```python
from build123d import *

# Parameters (mm, degrees)
SKETCH1_R               = 9.05
BOSS_EXTRUDE1_DEPTH     = 1.5
SKETCH2_R               = 7.83
BOSS_EXTRUDE2_DEPTH     = 11
CUT_EXTRUDE1_START      = -11
CUT_EXTRUDE1_DEPTH      = 11
SKETCH3_R               = 9.05
BOSS_EXTRUDE3_DEPTH     = 1.5
SKETCH5_R               = 6
BOSS_EXTRUDE4_DEPTH     = 9
SKETCH6_R               = 2.5
CUT_EXTRUDE2_DEPTH      = 27.321189183
CUT_EXTRUDE3_DEPTH      = 27.321189183
CUT_EXTRUDE3_DEPTH_BACK = 27.321189183
SKETCH7_R               = 1.5
FILLET1_R               = 0.2


with BuildPart() as part:
    # Sketch1 → Boss-Extrude1 (new body)
    with BuildSketch(Plane(origin=(0, 0, 0), x_dir=(1, 0, 0), z_dir=(0, 1, 0))):
        with Locations(Location((0, 0, 0), (0, 0, 270))):
            Circle(SKETCH1_R)
    extrude(amount=BOSS_EXTRUDE1_DEPTH)

    # Sketch2 → Boss-Extrude2 (add)
    with BuildSketch(Plane(origin=(0, 1.5, 0), x_dir=(1, 0, 0), z_dir=(0, 1, 0))):
        with Locations(Location((0, 0, 0), (0, 0, 270))):
            Circle(SKETCH2_R)
    extrude(amount=BOSS_EXTRUDE2_DEPTH)

    # Sketch4 → Cut-Extrude1 (cut)
    with BuildSketch(Plane(origin=(0, 12.5, 0), x_dir=(1, 0, 0), z_dir=(0, 1, 0)).offset(CUT_EXTRUDE1_START)):
        with BuildLine():
            Line((-1.095041255, 6.913818384), (-1.224881861, 7.733599707))
            ThreePointArc((-1.224881861, 7.733599707), (0, 7.83), (1.224881861, 7.733599707))
            Line((1.224881861, 7.733599707), (1.095041255, 6.913818384))
            ThreePointArc((1.095041255, 6.913818384), (0, 7), (-1.095041255, 6.913818384))
        make_face()
        with BuildLine():
            Line((3.177933498, 6.237045669), (3.554745613, 6.976581084))
            ThreePointArc((3.554745613, 6.976581084), (4.602358525, 6.334603066), (5.536646097, 5.536646097))
            Line((5.536646097, 5.536646097), (4.949747468, 4.949747468))
            ThreePointArc((4.949747468, 4.949747468), (4.114496766, 5.663118961), (3.177933498, 6.237045669))
        make_face()
        with BuildLine():
            Line((6.237045669, 3.177933498), (6.976581084, 3.554745613))
            ThreePointArc((6.976581084, 3.554745613), (7.446772523, 2.419603066), (7.733599707, 1.224881861))
            Line((7.733599707, 1.224881861), (6.913818384, 1.095041255))
            ThreePointArc((6.913818384, 1.095041255), (6.657395614, 2.163118961), (6.237045669, 3.177933498))
        make_face()
        with BuildLine():
            Line((6.913818384, -1.095041255), (7.733599707, -1.224881861))
            ThreePointArc((7.733599707, -1.224881861), (7.446772523, -2.419603066), (6.976581084, -3.554745613))
            Line((6.976581084, -3.554745613), (6.237045669, -3.177933498))
            ThreePointArc((6.237045669, -3.177933498), (6.657395614, -2.163118961), (6.913818384, -1.095041255))
        make_face()
        with BuildLine():
            Line((4.949747468, -4.949747468), (5.536646097, -5.536646097))
            ThreePointArc((5.536646097, -5.536646097), (4.602358525, -6.334603066), (3.554745613, -6.976581084))
            Line((3.554745613, -6.976581084), (3.177933498, -6.237045669))
            ThreePointArc((3.177933498, -6.237045669), (4.114496766, -5.663118961), (4.949747468, -4.949747468))
        make_face()
        with BuildLine():
            Line((1.095041255, -6.913818384), (1.224881861, -7.733599707))
            ThreePointArc((1.224881861, -7.733599707), (0, -7.83), (-1.224881861, -7.733599707))
            Line((-1.224881861, -7.733599707), (-1.095041255, -6.913818384))
            ThreePointArc((-1.095041255, -6.913818384), (0, -7), (1.095041255, -6.913818384))
        make_face()
        with BuildLine():
            Line((-3.177933498, -6.237045669), (-3.554745613, -6.976581084))
            ThreePointArc((-3.554745613, -6.976581084), (-4.602358525, -6.334603066), (-5.536646097, -5.536646097))
            Line((-5.536646097, -5.536646097), (-4.949747468, -4.949747468))
            ThreePointArc((-4.949747468, -4.949747468), (-4.114496766, -5.663118961), (-3.177933498, -6.237045669))
        make_face()
        with BuildLine():
            Line((-6.237045669, -3.177933498), (-6.976581084, -3.554745613))
            ThreePointArc((-6.976581084, -3.554745613), (-7.446772523, -2.419603066), (-7.733599707, -1.224881861))
            Line((-7.733599707, -1.224881861), (-6.913818384, -1.095041255))
            ThreePointArc((-6.913818384, -1.095041255), (-6.657395614, -2.163118961), (-6.237045669, -3.177933498))
        make_face()
        with BuildLine():
            Line((-6.913818384, 1.095041255), (-7.733599707, 1.224881861))
            ThreePointArc((-7.733599707, 1.224881861), (-7.446772523, 2.419603066), (-6.976581084, 3.554745613))
            Line((-6.976581084, 3.554745613), (-6.237045669, 3.177933498))
            ThreePointArc((-6.237045669, 3.177933498), (-6.657395614, 2.163118961), (-6.913818384, 1.095041255))
        make_face()
        with BuildLine():
            Line((-4.949747468, 4.949747468), (-5.536646097, 5.536646097))
            ThreePointArc((-5.536646097, 5.536646097), (-4.602358525, 6.334603066), (-3.554745613, 6.976581084))
            Line((-3.554745613, 6.976581084), (-3.177933498, 6.237045669))
            ThreePointArc((-3.177933498, 6.237045669), (-4.114496766, 5.663118961), (-4.949747468, 4.949747468))
        make_face()
    extrude(amount=CUT_EXTRUDE1_DEPTH, mode=Mode.SUBTRACT)

    # Sketch3 → Boss-Extrude3 (add)
    with BuildSketch(Plane(origin=(0, 12.5, 0), x_dir=(1, 0, 0), z_dir=(0, 1, 0))):
        with Locations(Location((0, 0, 0), (0, 0, 270))):
            Circle(SKETCH3_R)
    extrude(amount=BOSS_EXTRUDE3_DEPTH)

    # Sketch5 → Boss-Extrude4 (add)
    with BuildSketch(Plane(origin=(0, 14, 0), x_dir=(1, 0, 0), z_dir=(0, 1, 0))):
        with Locations(Location((0, 0, 0), (0, 0, 270))):
            Circle(SKETCH5_R)
    extrude(amount=BOSS_EXTRUDE4_DEPTH)

    # Sketch6 → Cut-Extrude2 (cut, through all)
    with BuildSketch(Plane(origin=(0, 23, 0), x_dir=(1, 0, 0), z_dir=(0, 1, 0))):
        with Locations(Location((0, 0, 0), (0, 0, 270))):
            Circle(SKETCH6_R)
    extrude(amount=-CUT_EXTRUDE2_DEPTH, mode=Mode.SUBTRACT)

    # Sketch7 → Cut-Extrude3 (cut, two sides: drawn at the far end of the back side and taken through both)
    with BuildSketch(Plane.XY.offset(-CUT_EXTRUDE3_DEPTH_BACK)):
        with Locations((0, 18)):
            Circle(SKETCH7_R)
    extrude(amount=CUT_EXTRUDE3_DEPTH + CUT_EXTRUDE3_DEPTH_BACK, mode=Mode.SUBTRACT)

    # Fillet1
    fillet1_edges = [part.edges().sort_by_distance(p)[0] for p in [
        (0, 14, -6),
        (0, 23, -6),
        (0, 0, -2.5),
        (0, 23, -2.5),
    ]]
    fillet(fillet1_edges, radius=FILLET1_R)


solid = part.part
```
Work out the finished part from the listing and answer in its coordinate system (mm). A direction names the side the tool comes from. Round coordinates to 2 decimals unless told otherwise and drop trailing zeros. Order: outer loops, then holes, each group sorted by start corner. A loop starts at its lowest first (then second) coordinate and runs counter-clockwise, first axis right, second up.
Q1. A cutting plane is placed at B-B, the plane y = 18. Determine the outline of the cut face in (x, z), then the cut area to 3 significant figures.
Solution:
outline: (-1.5, -5.81) - (-1.5, -2) arc R2.5 cw to (-1.5, 2) - (-1.5, 5.81) arc R6 ccw to start; (1.5, -5.81) arc R6 ccw to (1.5, 5.81) - (1.5, 2) arc R2.5 cw to (1.5, -2) - close
area: 71.9 mm2
Q2. Given pin 1 Ø4 at (x, y) = (0, 5) entering from -Z; pin 2 Ø3.5 at (x, y) = (0, 18) entering from -Z; pin 3 Ø2.5 at (x, y) = (0, 18) entering from +Z; pin 4 Ø1 at (y, z) = (10, -6.5) entering from +X, each flat-ended and moving along its own axis, determine where each tip first touches the part or whether it passes through.
Solution:
pin 1: stops at z = -7.73
pin 2: stops at z = -6
pin 3: passes through
pin 4: stops at x = 3.61
Q3. The mould has two halves that part along X. Classify faces 4 (the cylindrical face through (1.802, 18.44, 5.723)), 5 (the flat face through (-1.16, 6.92, -7.32)), 6 (the cylindrical face through (-6.345, 6.923, 4.588)): pulls with the +X half, pulls with the -X half, needs draft (parallel to the pull), parting line crosses it, or undercut.
Solution:
face 4: parting line crosses it
face 5: undercut
face 6: pulls with the -X half
Q4. A cutting plane is placed at A-A, the plane z = 0. Determine the outline of the cut face in (x, y), then the cut area to 3 significant figures.
Solution:
outline: (-9.05, 0) - (-2.7, 0) arc R0.2 ccw to (-2.5, 0.2) - (-2.5, 22.8) arc R0.2 ccw to (-2.7, 23) - (-5.8, 23) arc R0.2 ccw to (-6, 22.8) - (-6, 14.2) arc R0.2 cw to (-6.2, 14) - (-9.05, 14) - (-9.05, 12.5) - (-7.83, 12.5) - (-7.83, 1.5) - (-9.05, 1.5) - close; (2.5, 0.2) arc R0.2 ccw to (2.7, 0) - (9.05, 0) - (9.05, 1.5) - (7.83, 1.5) - (7.83, 12.5) - (9.05, 12.5) - (9.05, 14) - (6.2, 14) arc R0.2 cw to (6, 14.2) - (6, 22.8) arc R0.2 ccw to (5.8, 23) - (2.7, 23) arc R0.2 ccw to (2.5, 22.8) - close
area: 220 mm2
Q5. A cutting plane is placed at D-D, the plane y = 21.25. Determine the outline of the cut face in (x, z).
Solution:
outline: circle Ø12 at (0, 0); hole circle Ø5 at (0, 0)
Q6. Find the intervals of material crossed by line 1 along Z through (x, y) = (0, 14.75); line 2 along Z through (x, y) = (0, 5.25); line 3 along Y through (x, z) = (0, 4.5), in increasing order.
Solution:
line 1: z = -6 to -2.5, 2.5 to 6
line 2: z = -7 to -2.5, 2.5 to 7
line 3: y = 0 to 16.5, 19.5 to 23
Q7. A tool of negligible diameter and unlimited length cuts with its end or side. For faces 1 (the cylindrical face through (0, 7, 7)), 2 (the flat face through (-4.7, 1.5, -5.4)), 3 (the cylindrical face through (2.403, 6.923, 7.452)), from which of +Z, -Z, +X, -X, +Y, -Y can it reach the whole face along a straight path? Write none if from no direction.
Solution:
face 1: +Z
face 2: none
face 3: +Z, +X
Q8. A cutting plane is placed at C-C, the plane x = 0. Count the separate pieces of the cut face and the enclosed holes in it, then the cut area to 3 significant figures.
Solution:
separate pieces: 4
enclosed holes: 0
area: 180 mm2
